from build123d import *

# Parameters (mm, degrees)
BOSS_EXTRU_1_DEPTH      = 10
ESQUISSE2_R             = 3
ENL_V_MAT_EXTRU_1_DEPTH = 21
CHANFREIN1_SIZE         = 0.5
TROU_TARAUD_M41_D       = 3.3
TROU_TARAUD_M41_DEPTH   = 10.1
TROU_TARAUD_M41_TIP     = 0.991420021


with BuildPart() as part:
    # Esquisse1 → Boss.-Extru.1 (new body, symmetric)
    with BuildSketch(Plane.XY):
        Polygon((-16, 20), (16, 20), (16, 0), (11, 0), (11, 15), (-11, 15), (-11, 0), (-16, 0), align=None)
    extrude(amount=BOSS_EXTRU_1_DEPTH, both=True)

    # Esquisse2 → Enlèv. mat.-Extru.1 (cut, through all)
    with BuildSketch(Plane(origin=(0, 20, 0), x_dir=(1, 0, 0), z_dir=(0, 1, 0))):
        Circle(ESQUISSE2_R)
    extrude(amount=-ENL_V_MAT_EXTRU_1_DEPTH, mode=Mode.SUBTRACT)

    # Chanfrein1
    chanfrein1_edges = [part.edges().sort_by_distance(p)[0] for p in [
        (-3, 15, 0),
        (-3, 20, 0),
    ]]
    chamfer(chanfrein1_edges, length=CHANFREIN1_SIZE)

    # Trou taraudé M41
    with Locations(Plane.XZ):
        with Locations((13.5, 5), (-13.5, -5), (-13.5, 5), (13.5, -5)):
            Hole(TROU_TARAUD_M41_D / 2, depth=TROU_TARAUD_M41_DEPTH)
            with Locations((0, 0, -(TROU_TARAUD_M41_DEPTH + TROU_TARAUD_M41_TIP / 2))):  # 118° drill point
                Cone(0, TROU_TARAUD_M41_D / 2, TROU_TARAUD_M41_TIP, mode=Mode.SUBTRACT)


solid = part.part
Here's how the part is built. I have some questions about the finished solid (model axes, mm). A direction names the side the tool comes from. Coordinates: 2 decimals unless noted, no trailing zeros. Loops run counter-clockwise (first coordinate to the right, second up) from the corner with the lowest first, then second, coordinate; pieces in that order, holes last. Notation, with made-up numbers: (9, 79.5) -> (66, 79.5) arc R13 cw to (66, 101.5) -> close; hole circle Ø2 at (35, 31.25). An arc over 180 degrees is marked (long way). Use one line per item in the form item = value. Start each with the question number.
(1) On a 3-axis mill with a long thin cutter (end or side, diameter ignored), from which of +Z, -Z, +X, -X, +Y, -Y can I reach the whole of each face in a straight line? I mean faces 4 (the face through (11, 7, 0)), 5 (the face through (-4, 20, 0)), 6 (the face through (11.976, 5.121, -5.632)). Say none if no direction works.
(2) Will these pins go through, and if not, where does the flat tip stop? pin 1 (2 mm diameter, centred on x = 13.5, z = 5, fed in from -Y); pin 2 (2.5 mm diameter, centred on x = -13.5, z = -5, fed in from -Y); pin 3 (9.5 mm diameter, centred on x = 0, z = 0, fed in from -Y).
(3) We'd pull the mould along X, two halves only. Please class faces 1 (the face through (0, 17, 10)), 2 (the face through (0, 15, 5)), 3 (the face through (16, 10, 0)): pulls with the +X half, pulls with the -X half, needs draft (parallel to the pull), parting line crosses it, or undercut.
(4) If we section it at A-A (y = 8.5): Please give me the cut outline in (x, z), then the cut area to 3 significant figures.
(5) If we section it at B-B (z = 0): Please give me the cut outline in (x, y).
(6) If we section it at C-C (x = 0): Please give me the cut outline in (y, z).
(7) If we section it at D-D (y = 12.25): Please give me the cut outline in (x, z), then the cut area to 3 significant figures.
(8) Please list where these lines run through material, in increasing order: line 1 along X through (y, z) = (7.75, 5); line 2 along Z through (x, y) = (13.5, 3.25); line 3 along X through (y, z) = (18.6, 0).
Verdict:
q1.face_4 = +Z, -Z, -Y
q1.face_5 = +Z, -Z, +X, -X, +Y
q1.face_6 = -Y
q2.pin_1 = 10.49
q2.pin_2 = 10.34
q2.pin_3 = 15
q3.face_1 = needs draft
q3.face_2 = undercut
q3.face_3 = pulls with the +X half
q4.outline = (-16, -10) -> (-11, -10) -> (-11, 10) -> (-16, 10) -> close; (11, -10) -> (16, -10) -> (16, 10) -> (11, 10) -> close; hole circle Ø3.3 at (-13.5, -5); hole circle Ø3.3 at (-13.5, 5); hole circle Ø3.3 at (13.5, -5); hole circle Ø3.3 at (13.5, 5)
q4.area = 166 mm²
q5.outline = (-16, 0) -> (-11, 0) -> (-11, 15) -> (-3.5, 15) -> (-3, 15.5) -> (-3, 19.5) -> (-3.5, 20) -> (-16, 20) -> close; (3, 15.5) -> (3.5, 15) -> (11, 15) -> (11, 0) -> (16, 0) -> (16, 20) -> (3.5, 20) -> (3, 19.5) -> close
q6.outline = (15, -10) -> (20, -10) -> (20, -3.5) -> (19.5, -3) -> (15.5, -3) -> (15, -3.5) -> close; (15, 3.5) -> (15.5, 3) -> (19.5, 3) -> (20, 3.5) -> (20, 10) -> (15, 10) -> close
q7.outline = (-16, -10) -> (-11, -10) -> (-11, 10) -> (-16, 10) -> close; (11, -10) -> (16, -10) -> (16, 10) -> (11, 10) -> close
q7.area = 200 mm²
q8.line_1 = -16 to -15.15, -11.85 to -11, 11 to 11.85, 15.15 to 16
q8.line_2 = -10 to -6.65, -3.35 to 3.35, 6.65 to 10
q8.line_3 = -16 to -3, 3 to 16
